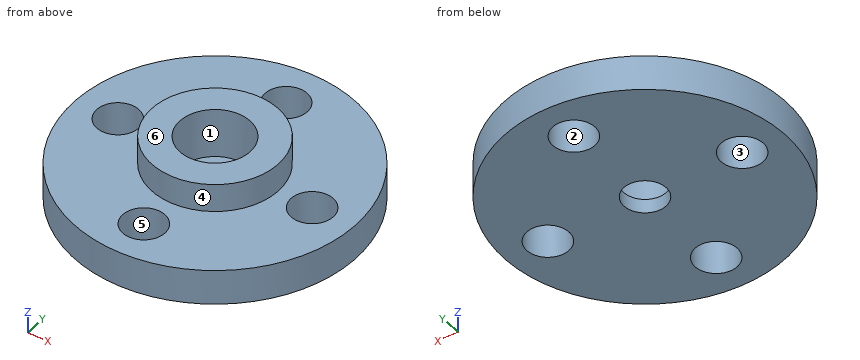
from build123d import *

# Parameters (mm, degrees)
F0_R      = 10
F1_DEPTH  = 2.5
F2_R      = 4.5
F2_R_2    = 2.5
F3_DEPTH  = 2
F3_FACE_R = 2.5
F4_DEPTH  = 1.5
F5_R      = 1.5
F6_DEPTH  = 25


with BuildPart() as f1:
    # F0 (on Top) → F1 (new body)
    with BuildSketch(Plane.XY):
        Circle(F0_R)
    extrude(amount=F1_DEPTH)

    # F2 (on face) → F3 (join)
    with BuildSketch(Plane.XY.offset(2.5)):
        Circle(F2_R)
        Circle(F2_R_2, mode=Mode.SUBTRACT)
    extrude(amount=F3_DEPTH)

    # F3_face (on face) → F4 (cut)
    with BuildSketch(Plane.XY.offset(2.5)):
        Circle(F3_FACE_R)
    extrude(amount=-F4_DEPTH, mode=Mode.SUBTRACT)

    # F5 (on face) → F6 (cut)
    with BuildSketch(Plane(origin=(0, 0, 0), x_dir=(1, 0, 0), z_dir=(0, 0, -1))):
        with Locations((-7, 0)):
            Circle(F5_R)
        with Locations((7, 0)):
            Circle(F5_R)
        with Locations((0, -7)):
            Circle(F5_R)
        with Locations((0, 7)):
            Circle(F5_R)
        Circle(F5_R)
    extrude(amount=-F6_DEPTH, mode=Mode.SUBTRACT)


solid = f1.part
Can you work these out from the model? Positions are in its coordinate system, mm. Face numbers are marked on the shaded views. A direction names the side the tool comes from. Round coordinates to 2 decimals unless told otherwise and drop trailing zeros. Loops run counter-clockwise (first coordinate to the right, second up) from the corner with the lowest first, then second, coordinate; pieces in that order, holes last. Notation, with made-up numbers: (87.25, 79.5) - (124.25, 79.5) arc R14 cw to (124.25, 97.5) - close; hole circle Ø5 at (36.25, -32.75). An arc over 180 degrees is marked (long way). Answer in a Markdown table with one row per item. Add a question column.
Q1. For pin 1 Ø1 at (y, z) = (4.5, 1.5) entering from -X; pin 2 Ø2 at (y, z) = (4.5, 1.5) entering from -X, each with a flat end and sliding along its axis, tell me the tip position at first contact or that it passes through.
Q2. I want a section at D-D on z = 1.8. List the corners of the cut face in (x, y) for me, and give its area (3 significant figures).
Q3. I want a section at B-B on y = 6. List the corners of the cut face in (x, z) for me, and give its area (3 significant figures).
Q4. I want a section at C-C on z = 4.1. List the corners of the cut face in (x, y) for me.
Q5. I want a section at A-A on x = 0. List the corners of the cut face in (y, z) for me, and give its area (3 significant figures).
Q6. I need wall thicknesses on L1, parallel to Y at x = 0, z = 0.9; L2, parallel to Y at x = 0, z = 1.8; L3, parallel to X at y = 1.25, z = 0.35. Which ranges of each line are inside material? Lowest first, please.
Q7. We'd pull the mould along Y, two halves only. Please class the marked faces 3, 4, 5 and 6: pulls with the +Y half, pulls with the -Y half, needs draft (parallel to the pull), parting line crosses it, or undercut.
Q8. Which directions (+Z, -Z, +X, -X, +Y, -Y) give clear straight access to the entire face, cutting with the end or side of a thin tool? Please do the marked faces 1 and 2.
A:
| question | item | result |
|---|---|---|
| 1 | pin 1 | x = -9.17 |
| 1 | pin 2 | x = -9.37 |
| 2 | outline | circle Ø20 at (0, 0); hole circle Ø3 at (-7, 0); hole circle Ø5 at (0, 0); hole circle Ø3 at (0, -7); hole circle Ø3 at (0, 7); hole circle Ø3 at (7, 0) |
| 2 | area | 266 mm^2 |
| 3 | outline | (-8, 0) - (-1.12, 0) - (-1.12, 2.5) - (-8, 2.5) - close; (1.12, 0) - (8, 0) - (8, 2.5) - (1.12, 2.5) - close |
| 3 | area | 34.4 mm^2 |
| 4 | outline | circle Ø9 at (0, 0); hole circle Ø5 at (0, 0) |
| 5 | outline | (-10, 0) - (-8.5, 0) - (-8.5, 2.5) - (-10, 2.5) - close; (-5.5, 0) - (-1.5, 0) - (-1.5, 1) - (-2.5, 1) - (-2.5, 4.5) - (-4.5, 4.5) - (-4.5, 2.5) - (-5.5, 2.5) - close; (1.5, 0) - (5.5, 0) - (5.5, 2.5) - (4.5, 2.5) - (4.5, 4.5) - (2.5, 4.5) - (2.5, 1) - (1.5, 1) - close; (8.5, 0) - (10, 0) - (10, 2.5) - (8.5, 2.5) - close |
| 5 | area | 32.5 mm^2 |
| 6 | L1 | -10 to -8.5, -5.5 to -1.5, 1.5 to 5.5, 8.5 to 10 |
| 6 | L2 | -10 to -8.5, -5.5 to -2.5, 2.5 to 5.5, 8.5 to 10 |
| 6 | L3 | -9.92 to -7.83, -6.17 to -0.83, 0.83 to 6.17, 7.83 to 9.92 |
| 7 | face 3 | undercut |
| 7 | face 4 | parting line crosses it |
| 7 | face 5 | undercut |
| 7 | face 6 | needs draft |
| 8 | face 1 | +Z |
| 8 | face 2 | +Z, -Z |
